The listing builds one solid part. Answer for the finished solid, in the listing's coordinates (mm). A direction names the side the tool comes from. Give positions to 0.01 mm unless a question says otherwise; leave off trailing zeros. Order: outer loops, then holes, each group sorted by start corner. A loop starts at its lowest first (then second) coordinate and runs counter-clockwise, first axis right, second up. Notation, with made-up numbers: (28.25, 0) - (83.25, 0) arc R32 ccw to (83.25, 35) - close; hole circle Ø6 at (2, 7). An arc over 180 degrees is marked (long way). Answer as a JSON object with one key per item and string values. Group by question number.
Q1. For faces 5 (the face through (-3, -13.5, 75)), 6 (the face through (-3, 13.5, 75)), 7 (the face through (-4, 12.5, 75)), 8 (the face through (-0.5, -0.1, 121.5)), determine the directions among +Z, -Z, +X, -X, +Y, -Y from which every point of the face is accessible in a straight line to the end or side of a thin tool.
Q2. The mould has two halves that part along Z. Classify faces 1 (the face through (-0.5, 0.1, 3.5)), 2 (the face through (-4, -12.5, 75)), 3 (the face through (-0.5, 0.1, 78.5)), 4 (the face through (-0.7, -1.2, 0)): released by +Z, released by -Z, zero draft, split by the parting line, or undercut.
Q3. A cutting plane is placed at A-A, the plane x = -4.5. Give the vertices of the cut face in (y, z), and give its area (3 significant figures).
Q4. Given pin 1 (2 mm diameter, centred on x = -2.5, z = 112, fed in from +Y); pin 2 (3 mm diameter, centred on y = -4.5, z = 26.5, fed in from -X); pin 3 (0.5 mm diameter, centred on x = -0.5, z = 139, fed in from -Y); pin 4 (4 mm diameter, centred on x = -3.5, y = -9.5, fed in from +Z), each flat-ended and moving along its own axis, determine where each tip first touches the part or whether it passes through.
Q5. A cutting plane is placed at D-D, the plane y = 10.5. Give the vertices of the cut face in (x, z), and give its area (3 significant figures).
Q6. A cutting plane is placed at C-C, the plane y = 1. Give the vertices of the cut face in (x, z), and give its area (3 significant figures).
Q7. A cutting plane is placed at B-B, the plane z = 100. Give the vertices of the cut face in (x, y).
Q8. Consider line 1 (Y direction, x = -4.5, z = 99.5); line 2 (Y direction, x = -6.75, z = 132.5); line 3 (X direction, y = 5, z = 71). Determine where each line is inside the solid, lowest interval first.
from build123d import *

# Parameters (mm, degrees)
EXTRUDE_THIN1_DEPTH = 449.2625
CUT_EXTRUDE1_START  = -8.5
CUT_EXTRUDE1_DEPTH  = 9.5
LPATTERN1_COUNT     = 18
LPATTERN1_PITCH     = 25
FILLET1_R           = 0.5
SKETCH5_W           = 23.532863881
SKETCH5_H           = 44.509442227
CUT_EXTRUDE2_DEPTH  = 296.8625


with BuildPart() as part:
    # Sketch3 → Extrude-Thin1 (new body)
    with BuildSketch(Plane.XY):
        Polygon((-6.5, 17.5), (-6.5, 13.5), (0, 13.5), (0, -13.5), (-6.5, -13.5), (-6.5, -17.5), (-7.5, -17.5), (-7.5, -12.5), (-1, -12.5), (-1, 12.5), (-7.5, 12.5), (-7.5, 17.5), align=None)
    extrude(amount=EXTRUDE_THIN1_DEPTH)

    # Sketch4 → Cut-Extrude1 (cut)
    with BuildSketch(Plane(origin=(0, 0, 0), x_dir=(0, 0, -1), z_dir=(1, 0, 0)).offset(CUT_EXTRUDE1_START)):
        with BuildLine():
            Line((-6.65, -3.15), (-18.35, -3.15))
            ThreePointArc((-18.35, -3.15), (-21.5, 0), (-18.35, 3.15))
            Line((-18.35, 3.15), (-6.65, 3.15))
            ThreePointArc((-6.65, 3.15), (-3.5, 0), (-6.65, -3.15))
        make_face()
    cut_extrude1 = extrude(amount=CUT_EXTRUDE1_DEPTH, mode=Mode.SUBTRACT)

    # LPattern1: Cut-Extrude1 ×18
    with Locations(*[(0, 0, i * LPATTERN1_PITCH) for i in range(1, LPATTERN1_COUNT)]):
        add(cut_extrude1, mode=Mode.SUBTRACT)

    # Fillet1
    fillet1_edges = [part.edges().sort_by_distance(p)[0] for p in [
        (-6.5, 13.5, 224.63125),
        (0, 13.5, 224.63125),
        (0, -13.5, 224.63125),
        (-6.5, -13.5, 224.63125),
        (-7.5, -12.5, 224.63125),
        (-1, -12.5, 224.63125),
        (-1, 12.5, 224.63125),
        (-7.5, 12.5, 224.63125),
    ]]
    fillet(fillet1_edges, radius=FILLET1_R)

    # Sketch5 → Cut-Extrude2 (cut)
    with BuildSketch(Plane.XY.offset(449.2625)):
        with Locations((-4.42532449, -0.836961712)):
            Rectangle(SKETCH5_W, SKETCH5_H)
    extrude(amount=-CUT_EXTRUDE2_DEPTH, mode=Mode.SUBTRACT)


solid = part.part
Reply:
{
 "1": {"face 5": "+Z, -Z, +X, -Y", "face 6": "+Z, -Z, +X, +Y", "face 7": "+Z, -Z, -X", "face 8": "+X, -X"},
 "2": {"face 1": "undercut", "face 2": "zero draft", "face 3": "undercut", "face 4": "released by -Z"},
 "3": {"outline": "(-13.5, 0) - (-12.5, 0) - (-12.5, 152.4) - (-13.5, 152.4) - close; (12.5, 0) - (13.5, 0) - (13.5, 152.4) - (12.5, 152.4) - close", "area": "305 mm^2"},
 "4": {"pin 1": "stops at y = 13.5", "pin 2": "stops at x = -1", "pin 3": "stops at y = -13.5", "pin 4": "passes through"},
 "5": {"outline": "(-1, 0) - (0, 0) - (0, 152.4) - (-1, 152.4) - close", "area": "152 mm^2"},
 "6": {"outline": "(-1, 0) - (0, 0) - (0, 3.66) - (-1, 3.66) - close; (-1, 21.34) - (0, 21.34) - (0, 28.66) - (-1, 28.66) - close; (-1, 46.34) - (0, 46.34) - (0, 53.66) - (-1, 53.66) - close; (-1, 71.34) - (0, 71.34) - (0, 78.66) - (-1, 78.66) - close; (-1, 96.34) - (0, 96.34) - (0, 103.66) - (-1, 103.66) - close; (-1, 121.34) - (0, 121.34) - (0, 128.66) - (-1, 128.66) - close; (-1, 146.34) - (0, 146.34) - (0, 152.4) - (-1, 152.4) - close", "area": "46.4 mm^2"},
 "7": {"outline": "(-7.5, -17.5) - (-6.5, -17.5) - (-6.5, -14) arc R0.5 cw to (-6, -13.5) - (-0.5, -13.5) arc R0.5 ccw to (0, -13) - (0, 13) arc R0.5 ccw to (-0.5, 13.5) - (-6, 13.5) arc R0.5 cw to (-6.5, 14) - (-6.5, 17.5) - (-7.5, 17.5) - (-7.5, 13) arc R0.5 ccw to (-7, 12.5) - (-1.5, 12.5) arc R0.5 cw to (-1, 12) - (-1, -12) arc R0.5 cw to (-1.5, -12.5) - (-7, -12.5) arc R0.5 ccw to (-7.5, -13) - close"},
 "8": {"line 1": "y = -13.5 to -12.5, 12.5 to 13.5", "line 2": "y = -17.5 to -12.5, 12.5 to 17.5", "line 3": "x = -1 to 0"}
}
